Read the model definition and answer for the solid it produces. Units are mm, in the model's axes. A direction names the side the tool comes from. Coordinates: 2 decimals unless noted, no trailing zeros. Loops run counter-clockwise (first coordinate to the right, second up) from the corner with the lowest first, then second, coordinate; pieces in that order, holes last. Notation, with made-up numbers: (38, 73) -> (59, 73) arc R21 ccw to (59, 104) -> close; hole circle Ø11 at (1, 44.25). An arc over 180 degrees is marked (long way). Answer as a JSON object with one key per item and string values. Group by question number.
1) Section B-B, the plane x = 15.5 is taken. Give the vertices of the cut face in (y, z), plus the area to 3 significant figures.
2) Determine the mould class of faces 1 (the face through (2.281, -13.194, 6.084)), 2 (the face through (48.728, -4, 6)), 3 (the face through (25, -8, 12)) for opening direction Y: released by +Y, released by -Y, zero draft, split by the parting line, or undercut.
3) Flat-ended cylindrical pins translate along their axes: P1, Ø0.8, axis at y = -4.5, z = 6, coming from the -X side; P2, Ø1.7, axis at y = -11, z = 8, coming from the -X side; P3, Ø6, axis at x = 13.5, z = 5, coming from the +Y side. Find the tip coordinate at first contact, or state that the pin passes through.
4) Section A-A, the plane z = 2.25 is taken. Give the vertices of the cut face in (x, y) (1 decimal).
5) Which of the six approach directions +Z, -Z, +X, -X, +Y, -Y give full straight-line access (tool end or side, diameter ignored) to faces 4 (the face through (12, -2.34, 6)), 5 (the face through (51.228, -13, 6)), 6 (the face through (50, -10.6, 6)), 7 (the face through (46, -12.625, 6))?
6) Consider probe 1 along X at (y, z) = (-7.75, 8); probe 2 along X at (y, z) = (-13, 3.5); probe 3 along X at (y, z) = (-11.25, 10.5). Determine where each line is inside the solid, lowest interval first. Write a range as [from, to].
7) Section C-C, the plane y = -7 is taken. Give the vertices of the cut face in (x, z), plus the area to 3 significant figures.
Autodesk Inventor part; units mm, degrees
ref_plane "YZ Plane" through (0, 0, 0) normal (1, 0, 0) x (0, 1, 0)
ref_plane "XZ Plane" through (0, 0, 0) normal (0, 1, 0) x (-1, 0, 0)
ref_plane "XY Plane" through (0, 0, 0) normal (0, 0, 1) x (1, 0, 0)
sketch "Sketch5" plane through (0, 0, 0) normal (0, 0, 1) x (1, 0, 0)
  line L0 (51.2279, -15.6) -> (51.2279, -10.6)
  line L1 (51.2279, -10.6) -> (48.7279, -10.6)
  line L2 (48.7279, -10.6) -> (48.7279, -12.625)
  line L3 (42.7279, -12.625) -> (42.7279, -2.975)
  line L4 (48.7279, -2.975) -> (48.7279, -5)
  line L5 (48.7279, -5) -> (51.2279, -5)
  line L6 (51.2279, -5) -> (51.2279, 0)
  line L7 (42.7279, -2.975) -> (48.7279, -2.975)
  line L8 (42.7279, -12.625) -> (48.7279, -12.625)
  line L9 (51.2279, -15.6) -> (43.6357, -15.6)
  line L10 (39.8786, -15.6) -> (43.6357, -15.6)
  line L11 (0, -15.6) -> (39.8786, -15.6)
  line L12 (36.9909, 0) -> (51.2279, 0)
  line L13 (0, -15.6) -> (0, -5.4692)
  line L14 (36.9909, 0) -> (31.0226, 0)
  line L15 (34.0067, 0) -> (20.7329, -2.3405)
  line L16 (0, -5.4692) -> (0, -2.3405)
  line L17 (0, -2.3405) -> (20.7329, -2.3405)
  point P0 (0, 0)
  point P1 (44.1094, 0)
  dimension "d41" = 6
  dimension "d50" = 2.5
  dimension "d87" = 5.6
  dimension "d88" = 9.65
  dimension "d122" = 14.237
  dimension "d123" = 2.975
  dimension "d132" = 10
extrude "Extrusion2" add sketch "Sketch5" along normal blind 12
sketch "Sketch11" plane through (0, 0, 12) normal (0, 0, 1) x (1, 0, 0)
  line L0 (42.7279, -2.975) -> (48.7279, -2.975)
  circle A0 centre (42.7279, -2.975) radius 0.5
  line L1 (42.7279, -12.625) -> (42.7279, -2.975)
  circle A1 centre (42.7279, -12.625) radius 0.5
  line L2 (48.7279, -12.625) -> (42.7279, -12.625)
  circle A2 centre (48.7279, -12.625) radius 0.5
  line L3 (48.7279, -2.975) -> (48.7279, -5)
  circle A3 centre (48.7279, -2.975) radius 0.5
  point P0 (0, 0)
  dimension "d99" = 1
  dimension "d100" = 1
  dimension "d101" = 1
  dimension "d102" = 1
extrude "Extrusion7" cut sketch "Sketch11" against normal through all
fillet "Rundung4" radius 8 1 edges at (0, -15.6, 6)
sketch "Skizze13" plane through (0, 0, 0) normal (-1, 0, 0) x (0, 0, 1)
  point P0 (0, 0)
fillet "Rundung7" radius 4 1 edges at (0, -2.3405, 6)
equation "\"l1\" = 8"
properties part number "Maria_Greifer_Dreieck2_3D-Druck"
Determined:
{
 "1": {"outline": "(-15.6, 0) -> (-2.34, 0) -> (-2.34, 12) -> (-15.6, 12) -> close", "area": "159 mm²"},
 "2": {"face 1": "released by -Y", "face 2": "undercut", "face 3": "zero draft"},
 "3": {"P1": "x = 0.27", "P2": "x = 0.42", "P3": "y = -2.34"},
 "4": {"outline": "(0, -7.6) arc R8 ccw to (8, -15.6) -> (51.2, -15.6) -> (51.2, -10.6) -> (48.7, -10.6) -> (48.7, -12.1) arc R0.5 cw (long way) to (48.2, -12.6) -> (43.2, -12.6) arc R0.5 cw (long way) to (42.7, -12.1) -> (42.7, -3.5) arc R0.5 cw (long way) to (43.2, -3) -> (48.2, -3) arc R0.5 cw (long way) to (48.7, -3.5) -> (48.7, -5) -> (51.2, -5) -> (51.2, 0) -> (34, 0) -> (20.7, -2.3) -> (4, -2.3) arc R4 ccw to (0, -6.3) -> close"},
 "5": {"face 4": "+Z, -Z, -X, +Y", "face 5": "+Z, -Z, +X, +Y, -Y", "face 6": "+Z, -Z, +X", "face 7": "+Z, -Z"},
 "6": {"probe 1": "[0, 42.73]", "probe 2": "[2.1, 42.4], [43.06, 48.4], [49.06, 51.23]", "probe 3": "[0.88, 42.73], [48.73, 51.23]"},
 "7": {"outline": "(0, 0) -> (42.73, 0) -> (42.73, 12) -> (0, 12) -> close", "area": "513 mm²"}
}
